```python
from build123d import *

# Parameters (mm, degrees)
SKETCH1_R           = 1.625
SKETCH1_R_2         = 1.5
SKETCH1_R_3         = 30
BOSS_EXTRUDE1_DEPTH = 2


with BuildPart() as part:
    # Sketch1 → Boss-Extrude1 (new body)
    with BuildSketch(Plane(origin=(0, 3.76, 0), x_dir=(1, 0, 0), z_dir=(0, 1, 0))):
        with BuildLine():
            Line((-17.763717472, -58.375), (17.763717472, -58.375))
            ThreePointArc((17.763717472, -58.375), (29.244220443, -56.091385975), (38.976920908, -49.588203436))
            Line((38.976920908, -49.588203436), (57.136192155, -31.428932188))
            ThreePointArc((57.136192155, -31.428932188), (60.380425644, -29.261204675), (64.207259967, -28.5))
            Line((64.207259967, -28.5), (85.25, -28.5))
            Line((85.25, -28.5), (90.25, -23.5))
            Line((90.25, -23.5), (90.25, 23.5))
            Line((90.25, 23.5), (85.25, 28.5))
            Line((85.25, 28.5), (64.207259967, 28.5))
            ThreePointArc((64.207259967, 28.5), (60.380425644, 29.261204675), (57.136192155, 31.428932188))
            Line((57.136192155, 31.428932188), (38.976920908, 49.588203436))
            ThreePointArc((38.976920908, 49.588203436), (29.244220443, 56.091385975), (17.763717472, 58.375))
            Line((17.763717472, 58.375), (-17.763717472, 58.375))
            ThreePointArc((-17.763717472, 58.375), (-29.244220443, 56.091385975), (-38.976920908, 49.588203436))
            Line((-38.976920908, 49.588203436), (-57.136192155, 31.428932188))
            ThreePointArc((-57.136192155, 31.428932188), (-60.380425644, 29.261204675), (-64.207259967, 28.5))
            Line((-64.207259967, 28.5), (-85.25, 28.5))
            Line((-85.25, 28.5), (-90.25, 23.5))
            Line((-90.25, 23.5), (-90.25, -23.5))
            Line((-90.25, -23.5), (-85.25, -28.5))
            Line((-85.25, -28.5), (-64.207259967, -28.5))
            ThreePointArc((-64.207259967, -28.5), (-60.380425644, -29.261204675), (-57.136192155, -31.428932188))
            Line((-57.136192155, -31.428932188), (-38.976920908, -49.588203436))
            ThreePointArc((-38.976920908, -49.588203436), (-29.244220443, -56.091385975), (-17.763717472, -58.375))
        make_face()
        with Locations((31.996581849, 46.845824254)):
            Circle(SKETCH1_R, mode=Mode.SUBTRACT)
        with Locations((31.996581849, -46.845824254)):
            Circle(SKETCH1_R, mode=Mode.SUBTRACT)
        with Locations((-31.996581849, 46.845824254)):
            Circle(SKETCH1_R, mode=Mode.SUBTRACT)
        with Locations((58.5, -16.625)):
            Circle(SKETCH1_R_2, mode=Mode.SUBTRACT)
        with Locations((-58.5, 16.625)):
            Circle(SKETCH1_R_2, mode=Mode.SUBTRACT)
        with Locations((-58.5, -16.625)):
            Circle(SKETCH1_R_2, mode=Mode.SUBTRACT)
        with Locations((58.5, 16.625)):
            Circle(SKETCH1_R_2, mode=Mode.SUBTRACT)
        with Locations((-83.5, 16.625)):
            Circle(SKETCH1_R_2, mode=Mode.SUBTRACT)
        with Locations((-83.5, -16.625)):
            Circle(SKETCH1_R_2, mode=Mode.SUBTRACT)
        with Locations((83.5, -16.625)):
            Circle(SKETCH1_R_2, mode=Mode.SUBTRACT)
        with Locations((83.5, 16.625)):
            Circle(SKETCH1_R_2, mode=Mode.SUBTRACT)
        Circle(SKETCH1_R_3, mode=Mode.SUBTRACT)
        with Locations((46.845824254, 31.996581849)):
            Circle(SKETCH1_R, mode=Mode.SUBTRACT)
        with Locations((46.845824254, -31.996581849)):
            Circle(SKETCH1_R, mode=Mode.SUBTRACT)
        with Locations((-46.845824254, 31.996581849)):
            Circle(SKETCH1_R, mode=Mode.SUBTRACT)
        with Locations((-46.845824254, -31.996581849)):
            Circle(SKETCH1_R, mode=Mode.SUBTRACT)
        with Locations((-31.996581849, -46.845824254)):
            Circle(SKETCH1_R, mode=Mode.SUBTRACT)
        with BuildLine():
            Line((-15.875, -46.375), (-15.875, -41.375))
            ThreePointArc((-15.875, -41.375), (-14.849873734, -38.900126266), (-12.375, -37.875))
            Line((-12.375, -37.875), (12.375, -37.875))
            ThreePointArc((12.375, -37.875), (14.849873734, -38.900126266), (15.875, -41.375))
            Line((15.875, -41.375), (15.875, -46.375))
            ThreePointArc((15.875, -46.375), (14.849873734, -48.849873734), (12.375, -49.875))
            Line((12.375, -49.875), (-12.375, -49.875))
            ThreePointArc((-12.375, -49.875), (-14.849873734, -48.849873734), (-15.875, -46.375))
        make_face(mode=Mode.SUBTRACT)
        with BuildLine():
            Line((15.875, 46.375), (15.875, 41.375))
            ThreePointArc((15.875, 41.375), (14.849873734, 38.900126266), (12.375, 37.875))
            Line((12.375, 37.875), (-12.375, 37.875))
            ThreePointArc((-12.375, 37.875), (-14.849873734, 38.900126266), (-15.875, 41.375))
            Line((-15.875, 41.375), (-15.875, 46.375))
            ThreePointArc((-15.875, 46.375), (-14.849873734, 48.849873734), (-12.375, 49.875))
            Line((-12.375, 49.875), (12.375, 49.875))
            ThreePointArc((12.375, 49.875), (14.849873734, 48.849873734), (15.875, 46.375))
        make_face(mode=Mode.SUBTRACT)
        with BuildLine():
            Line((-43.5, -15.875), (-48.5, -15.875))
            ThreePointArc((-48.5, -15.875), (-50.974873734, -14.849873734), (-52, -12.375))
            Line((-52, -12.375), (-52, 12.375))
            ThreePointArc((-52, 12.375), (-50.974873734, 14.849873734), (-48.5, 15.875))
            Line((-48.5, 15.875), (-43.5, 15.875))
            ThreePointArc((-43.5, 15.875), (-41.025126266, 14.849873734), (-40, 12.375))
            Line((-40, 12.375), (-40, -12.375))
            ThreePointArc((-40, -12.375), (-41.025126266, -14.849873734), (-43.5, -15.875))
        make_face(mode=Mode.SUBTRACT)
        with BuildLine():
            Line((-32.438523587, -28.902989681), (-28.902989681, -32.438523587))
            ThreePointArc((-28.902989681, -32.438523587), (-28.170756634, -34.20629054), (-28.902989681, -35.974057493))
            Line((-28.902989681, -35.974057493), (-35.266950712, -42.338018524))
            ThreePointArc((-35.266950712, -42.338018524), (-37.034717665, -43.070251571), (-38.802484618, -42.338018524))
            Line((-38.802484618, -42.338018524), (-42.338018524, -38.802484618))
            ThreePointArc((-42.338018524, -38.802484618), (-43.070251571, -37.034717665), (-42.338018524, -35.266950712))
            Line((-42.338018524, -35.266950712), (-35.974057493, -28.902989681))
            ThreePointArc((-35.974057493, -28.902989681), (-34.20629054, -28.170756634), (-32.438523587, -28.902989681))
        make_face(mode=Mode.SUBTRACT)
        with BuildLine():
            Line((32.438523587, 28.902989681), (28.902989681, 32.438523587))
            ThreePointArc((28.902989681, 32.438523587), (28.170756634, 34.20629054), (28.902989681, 35.974057493))
            Line((28.902989681, 35.974057493), (35.266950712, 42.338018524))
            ThreePointArc((35.266950712, 42.338018524), (37.034717665, 43.070251571), (38.802484618, 42.338018524))
            Line((38.802484618, 42.338018524), (42.338018524, 38.802484618))
            ThreePointArc((42.338018524, 38.802484618), (43.070251571, 37.034717665), (42.338018524, 35.266950712))
            Line((42.338018524, 35.266950712), (35.974057493, 28.902989681))
            ThreePointArc((35.974057493, 28.902989681), (34.20629054, 28.170756634), (32.438523587, 28.902989681))
        make_face(mode=Mode.SUBTRACT)
        with BuildLine():
            Line((28.902989681, -32.438523587), (32.438523587, -28.902989681))
            ThreePointArc((32.438523587, -28.902989681), (34.20629054, -28.170756634), (35.974057493, -28.902989681))
            Line((35.974057493, -28.902989681), (42.338018524, -35.266950712))
            ThreePointArc((42.338018524, -35.266950712), (43.070251571, -37.034717665), (42.338018524, -38.802484618))
            Line((42.338018524, -38.802484618), (38.802484618, -42.338018524))
            ThreePointArc((38.802484618, -42.338018524), (37.034717665, -43.070251571), (35.266950712, -42.338018524))
            Line((35.266950712, -42.338018524), (28.902989681, -35.974057493))
            ThreePointArc((28.902989681, -35.974057493), (28.170756634, -34.20629054), (28.902989681, -32.438523587))
        make_face(mode=Mode.SUBTRACT)
        with BuildLine():
            Line((-28.902989681, 32.438523587), (-32.438523587, 28.902989681))
            ThreePointArc((-32.438523587, 28.902989681), (-34.20629054, 28.170756634), (-35.974057493, 28.902989681))
            Line((-35.974057493, 28.902989681), (-42.338018524, 35.266950712))
            ThreePointArc((-42.338018524, 35.266950712), (-43.070251571, 37.034717665), (-42.338018524, 38.802484618))
            Line((-42.338018524, 38.802484618), (-38.802484618, 42.338018524))
            ThreePointArc((-38.802484618, 42.338018524), (-37.034717665, 43.070251571), (-35.266950712, 42.338018524))
            Line((-35.266950712, 42.338018524), (-28.902989681, 35.974057493))
            ThreePointArc((-28.902989681, 35.974057493), (-28.170756634, 34.20629054), (-28.902989681, 32.438523587))
        make_face(mode=Mode.SUBTRACT)
        with BuildLine():
            Line((43.5, 15.875), (48.5, 15.875))
            ThreePointArc((48.5, 15.875), (50.974873734, 14.849873734), (52, 12.375))
            Line((52, 12.375), (52, -12.375))
            ThreePointArc((52, -12.375), (50.974873734, -14.849873734), (48.5, -15.875))
            Line((48.5, -15.875), (43.5, -15.875))
            ThreePointArc((43.5, -15.875), (41.025126266, -14.849873734), (40, -12.375))
            Line((40, -12.375), (40, 12.375))
            ThreePointArc((40, 12.375), (41.025126266, 14.849873734), (43.5, 15.875))
        make_face(mode=Mode.SUBTRACT)
    extrude(amount=-BOSS_EXTRUDE1_DEPTH)


solid = part.part
```
Verification items for the finished model (mm, model axes). A direction names the side the tool comes from. Coordinates: 2 decimals unless noted, no trailing zeros. Loops run counter-clockwise (first coordinate to the right, second up) from the corner with the lowest first, then second, coordinate; pieces in that order, holes last. Notation, with made-up numbers: (-6, 49) - (21, 49) arc R23 ccw to (21, 87) - close; hole circle Ø7 at (20, 61.5). An arc over 180 degrees is marked (long way). Put each result on its own line as item: value.
Item 1: Set-up check for faces 4 (the face through (14.88, 2.77, -38.93)), 5 (the face through (87.715, 2.774, 26.035)): record each of +Z, -Z, +X, -X, +Y, -Y from which the full face is reachable in a straight line by a thin tool's end or side.
Conclusion:
face 4: +Y, -Y
face 5: +Z, +X, +Y, -Y
Item 2: Draft check along X on faces 1 (the face through (29.396, 2.774, -56.028)), 2 (the face through (-29.092, 2.774, -56.154)), 3 (the face through (32.13, 2.77, 39.2)). Enter one of: pulls with the +X half, pulls with the -X half, needs draft (parallel to the pull), parting line crosses it, or undercut.
Conclusion:
face 1: pulls with the +X half
face 2: pulls with the -X half
face 3: undercut
Item 3: Section check C-C (y = 3.1). Give the number of separate pieces and of enclosed holes in the cut face, then the cut area to 3 significant figures.
Conclusion:
separate pieces: 1
enclosed holes: 25
area: 10,600 mm2
Item 4: Scan lines: line 1 along Z through (x, y) = (-0.5, 3.1) (3 decimals); line 2 along Z through (x, y) = (83.5, 2.3) (3 decimals); line 3 along X through (y, z) = (3.4, 0.5). Record each from-to range of solid material in increasing order.
Conclusion:
line 1: z = -58.375 to -49.875, -37.875 to -29.996, 29.996 to 37.875, 49.875 to 58.375
line 2: z = -28.5 to -18.125, -15.125 to 15.125, 18.125 to 28.5
line 3: x = -90.25 to -52, -40 to -30, 30 to 40, 52 to 90.25
Item 5: Section check D-D (x = 72). Enter the section's corners in (y, z).
Conclusion:
outline: (1.76, -28.5) - (3.76, -28.5) - (3.76, 28.5) - (1.76, 28.5) - close
Item 6: Section check A-A (z = 0). Enter the section's corners in (x, y), then the cut area to 3 significant figures.
Conclusion:
outline: (-90.25, 1.76) - (-52, 1.76) - (-52, 3.76) - (-90.25, 3.76) - close; (-40, 1.76) - (-30, 1.76) - (-30, 3.76) - (-40, 3.76) - close; (30, 1.76) - (40, 1.76) - (40, 3.76) - (30, 3.76) - close; (52, 1.76) - (90.25, 1.76) - (90.25, 3.76) - (52, 3.76) - close
area: 193 mm2
Item 7: Gauge pin test, flat ends, axial feed: pin 1 Ø3.5 at (x, z) = (46.85, -32) entering from +Y; pin 2 Ø0.6 at (x, y) = (45.5, 3) entering from +Z; pin 3 Ø0.6 at (x, y) = (-75.5, 3) entering from +Z. Record the tip position at first contact, or that the pin passes through.
Conclusion:
pin 1: stops at y = 3.76
pin 2: stops at z = 43.37
pin 3: stops at z = 28.5
Item 8: Section check B-B (x = 1.5). Enter the section's corners in (y, z) (3 decimals).
Conclusion:
outline: (1.76, -58.375) - (3.76, -58.375) - (3.76, -49.875) - (1.76, -49.875) - close; (1.76, -37.875) - (3.76, -37.875) - (3.76, -29.962) - (1.76, -29.962) - close; (1.76, 29.962) - (3.76, 29.962) - (3.76, 37.875) - (1.76, 37.875) - close; (1.76, 49.875) - (3.76, 49.875) - (3.76, 58.375) - (1.76, 58.375) - close
